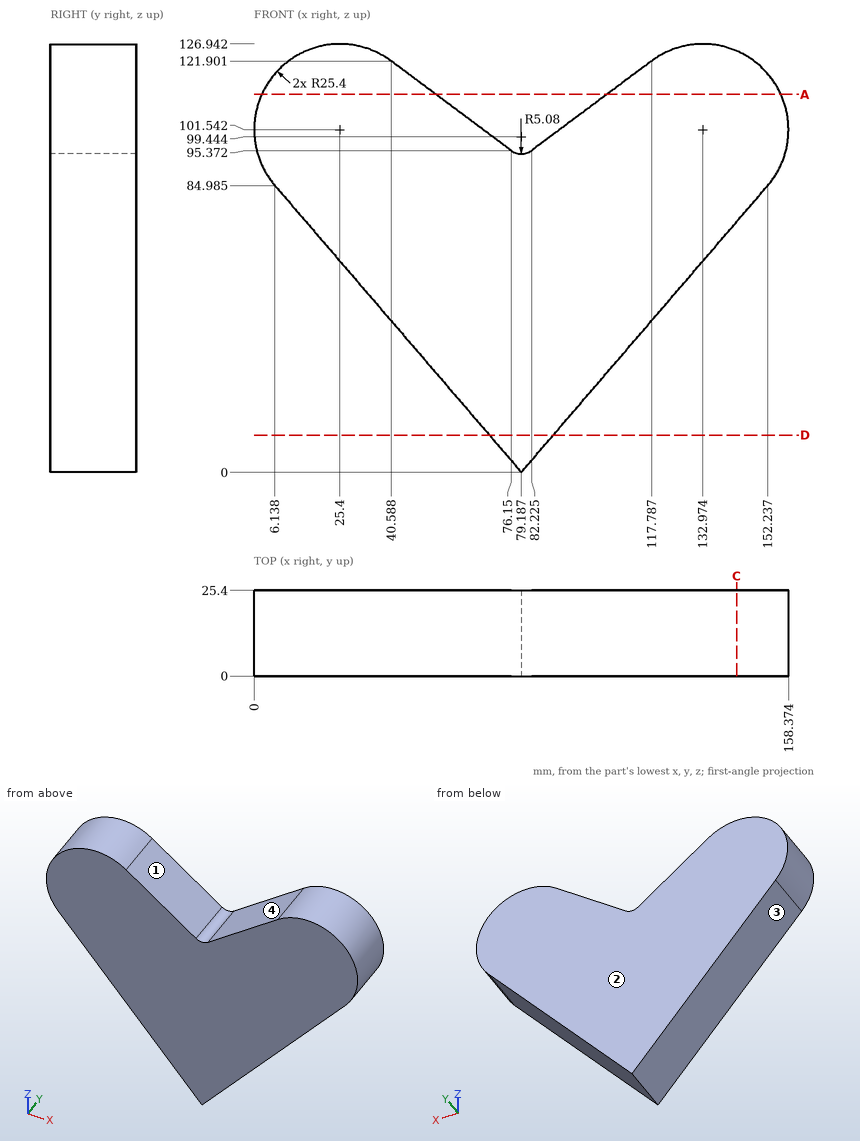
Input: dimensioned drawing with shaded views. Units: mm. Origin: part minimum x, y, z. Give positions to 0.01 mm unless a question says otherwise; leave off trailing zeros. Write each loop counter-clockwise with the first axis right and the second up, starting at its lowest first coordinate (ties: lowest second). Pieces come first, ordered by that corner, then holes. Notation, with made-up numbers: M -30.5,77 L -18.5,77 A9 ccw -18.5,93 Z; hole C -11.5,1 d4. An arc over 180 degrees is marked long. Return JSON: item names as keys, results as strings. Group by question number.
1) Pin query (flat end, axial travel): P1, Ø8, axis at x = 128, y = 3, coming from the +Z side; P2, Ø10, axis at y = 6.5, z = 16.5, coming from the -X side; P3, Ø4, axis at y = 17.5, z = 22, coming from the +X side (1 decimal). Return the tip coordinate at first contact, or that it passes through.
2) Cut plane A-A, the plane z = 112. Output: boundary loops of the cut face in (x, y) (1 decimal).
3) Material intervals for line 1 along X through (y, z) = (3.75, 119.5) (1 decimal); line 2 along Z through (x, y) = (150.5, 19.5) (1 decimal); line 3 along Z through (x, y) = (111, 19), sorted ascending. Write a range as [from, to].
4) Cut plane D-D, the plane z = 11. Output: boundary loops of the cut face in (x, y).
5) Pull-direction query (X, two-part tool) for the marked faces 1, 2, 3 and 4; classes: pulls with the +X half, pulls with the -X half, needs draft (parallel to the pull), parting line crosses it, or undercut.
6) Cut plane C-C, the plane x = 143. Output: boundary loops of the cut face in (y, z), plus the area to 3 significant figures.
Recorded:
{
 "1": {"P1": "stops at z = 126.92", "P2": "stops at x = 60.71", "P3": "stops at x = 99.8"},
 "2": {"outline": "M 2.3,0 L 53.9,0 L 53.9,25.4 L 2.3,25.4 Z; M 104.5,0 L 156.1,0 L 156.1,25.4 L 104.5,25.4 Z"},
 "3": {"line 1": "x = [7.4, 43.8], [114.6, 150.9]", "line 2": "z = [83, 119.9]", "line 3": "z = [37.01, 116.84]"},
 "4": {"outline": "M 69.73,0 L 88.64,0 L 88.64,25.4 L 69.73,25.4 Z"},
 "5": {"face 1": "undercut", "face 2": "needs draft", "face 3": "pulls with the -X half", "face 4": "undercut"},
 "6": {"outline": "M 0,74.24 L 25.4,74.24 L 25.4,124.88 L 0,124.88 Z", "area": "1,290 mm²"}
}
